Autodesk Inventor part; units mm, degrees
ref_plane "YZ Plane" through (0, 0, 0) normal (1, 0, 0) x (0, 1, 0)
ref_plane "XZ Plane" through (0, 0, 0) normal (0, 1, 0) x (-1, 0, 0)
ref_plane "XY Plane" through (0, 0, 0) normal (0, 0, 1) x (1, 0, 0)
sketch "Sketch1" plane through (0, 0, 0) normal (0, 0, 1) x (1, 0, 0)
  circle A0 centre (0, 0) radius 94.2975
  circle A1 centre (0, 0) radius 14.2875
  dimension "d0" = 188.595
  dimension "d1" = 28.575
extrude "Extrusion1" add sketch "Sketch1" along normal blind 6.35
sketch "Sketch2" plane through (0, 0, 6.35) normal (0, 0, 1) x (1, 0, 0)
  circle A0 centre (0, 0) radius 94.2975
  circle A1 centre (0, 0) radius 23.8125 construction
  line L0 (0, 0) -> (-11.9063, 20.6222) construction
  line L1 (0, 0) -> (0, 23.8125) construction
  circle A2 centre (-11.9063, 20.6222) radius 2.0193
  dimension "d4" = 47.625
  dimension "d5" = 30
  dimension "d6" = 4.0386
extrude "Extrusion2" cut sketch "Sketch2" against normal through all contours A2
pattern_circular "Circular Pattern1" count 6 over 360 about axis through (0, 0, -10) along (0, 0, 1) of "Extrusion2"
sketch "Sketch6" plane through (0, 0, 0) normal (0, 0, -1) x (-1, 0, 0)
  circle A0 centre (0, 0) radius 94.2975
  circle A1 centre (0, 0) radius 55.5625 construction
  line L0 (0, 0) -> (0, -55.5625) construction
  circle A2 centre (0, -55.5625) radius 2.4384
  circle A3 centre (0, 0) radius 14.2875
  line L1 (0, 0) -> (-39.2886, -39.2886) construction
  line L2 (0, 0) -> (39.2886, -39.2886) construction
  circle A4 centre (-39.2886, -39.2886) radius 2.4384
  circle A5 centre (39.2886, -39.2886) radius 2.4384
  dimension "d32" = 111.125
  dimension "d37" = 45
  dimension "d38" = 4.8768
extrude "Extrusion5" cut sketch "Sketch6" against normal up to next contours A2 | A4 | A5
pattern_circular "Circular Pattern4" count 2 over 360 about axis through (0, 0, -10) along (0, 0, 1) of "Extrusion5"
sketch "Sketch7" plane through (0, 0, 0) normal (0, 0, -1) x (-1, 0, 0)
  circle A0 centre (0, 0) radius 94.2975
  circle A1 centre (0, 0) radius 86.5188 construction
  circle A2 centre (0, -86.5188) radius 4.7625
  line L0 (0, -86.5188) -> (0, 0) construction
  dimension "d42" = 173.0375
  dimension "d43" = 9.525
extrude "Extrusion6" cut sketch "Sketch7" against normal through all contours A2
pattern_circular "Circular Pattern5" count 6 over 360 about axis through (0, 0, -10) along (0, 0, 1) of "Extrusion6"
sketch "Sketch8" plane through (0, 0, 0) normal (0, 0, -1) x (-1, 0, 0)
  circle A0 centre (0, 0) radius 94.2975
  arc A1 (-29.7576, 11.0702) -> (-29.7576, -11.0702) centre (0, 0) ccw
  arc A2 (-68.3565, 31.4575) -> (-68.3565, -31.4575) centre (0, 0) ccw
  line L0 (-59.413, 34.3021) -> (-32.5341, 18.7836)
  line L1 (-59.413, -34.3021) -> (-32.5341, -18.7836)
  line L2 (-27.4963, -15.875) -> (0, 0) construction
  line L3 (0, 0) -> (-27.4963, 15.875) construction
  line L4 (0, 0) -> (-75.2475, 0) construction
  line L5 (-65.1662, 37.6237) -> (-75.2475, 0) construction
  line L6 (-75.2475, 0) -> (-65.1662, -37.6237) construction
  arc A3 (-59.413, 34.3021) -> (-68.3565, 31.4575) centre (-62.588, 28.8029) ccw
  arc A4 (-29.7576, 11.0702) -> (-32.5341, 18.7836) centre (-35.7091, 13.2843) ccw
  arc A5 (-32.5341, -18.7836) -> (-29.7576, -11.0702) centre (-35.7091, -13.2843) ccw
  arc A6 (-68.3565, -31.4575) -> (-59.413, -34.3021) centre (-62.588, -28.8029) ccw
  dimension "d49" = 19.05
  dimension "d50" = 31.75
  dimension "d51" = 60
  dimension "d54" = 6.35
extrude "Extrusion7" cut sketch "Sketch8" against normal through all contours A1 A5 L1 A6 A2 A3 L0 A4
pattern_circular "Circular Pattern6" count 2 over 360 about axis through (0, 0, -10) along (0, 0, 1) of "Extrusion7"
sketch "Sketch9" plane through (0, 0, 0) normal (0, 0, -1) x (-1, 0, 0)
  arc A0 (29.7576, -11.0702) -> (29.7576, 11.0702) centre (0, 0) ccw
  circle A1 centre (0, 0) radius 94.2975
  circle A2 centre (0, 0) radius 69.85 construction
  line L0 (0, 0) -> (-34.925, 60.4919) construction
  line L1 (0, 0) -> (0, 69.85) construction
  circle A3 centre (-34.925, 60.4919) radius 12.7
  circle A4 centre (0, 0) radius 14.2875
  line L2 (0, 0) -> (34.925, 60.4919) construction
  circle A5 centre (34.925, 60.4919) radius 12.7
  dimension "d59" = 25.4
  dimension "d60" = 30
  dimension "d66" = 30
  dimension "d67" = 139.7
extrude "Extrusion8" cut sketch "Sketch9" against normal through all contours A3 | A5
pattern_circular "Circular Pattern7" count 2 over 360 about axis through (0, 0, -10) along (0, 0, 1) of "Extrusion8"
properties part number "FlyWheel_Base_Jan21" material "Aluminum-6061"
Verification items for the finished model (mm, model axes). A direction names the side the tool comes from. Round coordinates to 2 decimals unless told otherwise and drop trailing zeros. Order: outer loops, then holes, each group sorted by start corner. A loop starts at its lowest first (then second) coordinate and runs counter-clockwise, first axis right, second up.
1) Draft check along Y on faces 1 (the cylindrical face through (-64.583, 34.831, 3.131)), 2 (the flat face through (-46.16, -26.65, 3.13)), 3 (the flat face through (20, 1, 0)). Enter one of: +Y half, -Y half, draft (parallel to the pull), parting line (faces both ways), or undercut.
Geometry says:
face 1: undercut
face 2: undercut
face 3: draft
2) Tool access check on faces 4 (the cylindrical face through (64.583, -34.831, 3.131)), 5 (the flat face through (20, 1, 6.35)). Record the directions out of +Z, -Z, +X, -X, +Y, -Y that give a thin tool (end or side, any length) a straight path to the whole face; none if there is none.
Geometry says:
face 4: +Z, -Z
face 5: +Z, +X, -X, +Y, -Y
3) Material ranges on line 1 (Y direction, x = 0, z = 3); line 2 (X direction, y = -65.5, z = 0.75); line 3 (X direction, y = 9, z = 2.25), recorded low to high.
Geometry says:
line 1: y = -94.3 to -91.28, -81.76 to -58, -53.12 to -14.29, 14.29 to 53.12, 58 to 81.76, 91.28 to 94.3
line 2: x = -67.84 to -46.6, -23.25 to 23.25, 46.6 to 67.84
line 3: x = -93.87 to -74.71, -30.45 to -11.1, 11.1 to 30.45, 74.71 to 93.87
4) Cross-section at B-B, the plane y = 77.5. Record the cut outline in (x, z).
Geometry says:
outline: (-53.72, 0) - (53.72, 0) - (53.72, 6.35) - (-53.72, 6.35) - close
5) Cross-section at A-A, the plane x = 0. Record the cut outline in (y, z), plus the area to 3 significant figures.
Geometry says:
outline: (-94.3, 0) - (-91.28, 0) - (-91.28, 6.35) - (-94.3, 6.35) - close; (-81.76, 0) - (-58, 0) - (-58, 6.35) - (-81.76, 6.35) - close; (-53.12, 0) - (-14.29, 0) - (-14.29, 6.35) - (-53.12, 6.35) - close; (14.29, 0) - (53.12, 0) - (53.12, 6.35) - (14.29, 6.35) - close; (58, 0) - (81.76, 0) - (81.76, 6.35) - (58, 6.35) - close; (91.28, 0) - (94.3, 0) - (94.3, 6.35) - (91.28, 6.35) - close
area: 833 mm2
6) Cross-section at C-C, the plane z = 3.5. Give the number of separate pieces and of enclosed holes in the cut face, plus the area to 3 significant figures.
Geometry says:
separate pieces: 1
enclosed holes: 25
area: 19,800 mm2
7) Depth check by flat-ended pin: pin 1 (2 mm diameter, centred on y = -21, z = 5.5, fed in from -X); pin 2 (1 mm diameter, centred on y = 35, z = 4, fed in from +X); pin 3 (1.5 mm diameter, centred on x = -13, z = 4, fed in from +Y). Enter the tip coordinate at first touch or a pass-through.
Geometry says:
pin 1: stops at x = -92.15
pin 2: stops at x = 87.76
pin 3: stops at y = 93.5
